CAD build for the part. Positions are in the model's coordinates, mm. A direction names the side the tool comes from. Coordinates: 2 decimals unless noted, no trailing zeros. Order: outer loops, then holes, each group sorted by start corner. A loop starts at its lowest first (then second) coordinate and runs counter-clockwise, first axis right, second up. Notation, with made-up numbers: M 0.25,-23 L 33.25,-23 A29 cw 33.25,4 Z; hole C 47,21.25 d3. An arc over 180 degrees is marked long. Write item = value, one per line.
from build123d import *

# Parameters (mm, degrees)
F0_W     = 28
F0_H     = 18
F0_W_2   = 21.8
F0_H_2   = 11.8
F1_DEPTH = 7
F2_W     = 35.8
F2_H     = 18
F2_W_2   = 21.8
F2_H_2   = 11.8
F3_DEPTH = 2
F4_W     = 7
F4_H     = 3
F5_DEPTH = 31.901
F6_SIZE  = 1.5


with BuildPart() as f1:
    # F0 (on Right) → F1 (new body)
    with BuildSketch(Plane.YZ):
        Rectangle(F0_W, F0_H)
        Rectangle(F0_W_2, F0_H_2, mode=Mode.SUBTRACT)
    extrude(amount=-F1_DEPTH)

    # F2 (on face) → F3 (join)
    with BuildSketch(Plane.YZ):
        Rectangle(F2_W, F2_H)
        Rectangle(F2_W_2, F2_H_2, mode=Mode.SUBTRACT)
    extrude(amount=F3_DEPTH)

    # F4 (on face) → F5 (cut, through all)
    with BuildSketch(Plane(origin=(0, 14, 0), x_dir=(-1, 0, 0), z_dir=(0, 1, 0))):
        with Locations((3.5, 0)):
            Rectangle(F4_W, F4_H)
    extrude(amount=-F5_DEPTH, mode=Mode.SUBTRACT)

    # F6
    f6_edges = [f1.edges().sort_by_distance(p)[0] for p in [
        (2, 17.9, 0),
        (2, 0, 9),
        (2, -17.9, 0),
        (2, 0, -9),
        (2, 0, 5.9),
        (2, 10.9, 0),
        (2, 0, -5.9),
        (2, -10.9, 0),
    ]]
    chamfer(f6_edges, length=F6_SIZE)


solid = f1.part
(1) Pull direction Y, two halves, no side cores. Call faces 6 (the face through (-3, -14, 5)), 7 (the face through (0, -16, 0)), 8 (the face through (-3, -10.9, 3)): +Y half, -Y half, draft (parallel to the pull), parting line (faces both ways), or undercut.
Evaluation:
face_6 = -Y half
face_7 = draft
face_8 = undercut
(2) Wall check: line 1 (Z direction, x = -5.25, y = -11); line 2 (Z direction, x = -2.5, y = -5); line 3 (Y direction, x = -1.5, z = -4.25). Give the ranges that are in metal, low to high. Write a range as from..to.
Evaluation:
line_1 = -9..-1.5, 1.5..9
line_2 = -9..-5.9, 5.9..9
line_3 = -14..-10.9, 10.9..14
(3) Slice it at D-D, the plane z = 0. Write the cut outline in (x, y).
Evaluation:
outline = M 0,-17.9 L 0.5,-17.9 L 2,-16.4 L 2,-12.4 L 0.5,-10.9 L 0,-10.9 Z; M 0,10.9 L 0.5,10.9 L 2,12.4 L 2,16.4 L 0.5,17.9 L 0,17.9 Z
(4) Slice it at C-C, the plane y = 6.5. Write the cut outline in (x, z), then the cut area to 3 significant figures.
Evaluation:
outline = M -7,-9 L 0.5,-9 L 2,-7.5 L 2,-7.4 L 0.5,-5.9 L -7,-5.9 Z; M -7,5.9 L 0.5,5.9 L 2,7.4 L 2,7.5 L 0.5,9 L -7,9 Z
area = 51.3 mm²
(5) Pin check, flat tips, straight feed: pin 1 Ø1.5 at (x, z) = (-5, -1) entering from -Y; pin 2 Ø2 at (x, z) = (-3, -4.5) entering from +Y. Stop position of each tip, or through.
Evaluation:
pin_1 = -14
pin_2 = 14
(6) Slice it at B-B, the plane x = -5.25. Write the cut outline in (y, z).
Evaluation:
outline = M -14,-9 L 14,-9 L 14,-1.5 L 10.9,-1.5 L 10.9,-5.9 L -10.9,-5.9 L -10.9,-1.5 L -14,-1.5 Z; M -14,1.5 L -10.9,1.5 L -10.9,5.9 L 10.9,5.9 L 10.9,1.5 L 14,1.5 L 14,9 L -14,9 Z
(7) Tool access for faces 1 (the face through (-3, 0, 5.9)), 2 (the face through (-7, 0, 7)), 3 (the face through (1.3, -0.2, 6.7)), 4 (the face through (-3, 14, -5)), 5 (the face through (-3, -12, -1.5)): list every direction of +Z, -Z, +X, -X, +Y, -Y with a clear straight run to the whole face (end or side of a thin tool).
Evaluation:
face_1 = +X, -X
face_2 = +Z, -Z, -X, +Y, -Y
face_3 = +X
face_4 = +Z, -Z, -X, +Y
face_5 = -X, +Y, -Y
(8) Slice it at A-A, the plane z = -3.5. Write the cut outline in (x, y).
Evaluation:
outline = M -7,-14 L 0,-14 L 0,-17.9 L 0.5,-17.9 L 2,-16.4 L 2,-12.4 L 0.5,-10.9 L -7,-10.9 Z; M -7,10.9 L 0.5,10.9 L 2,12.4 L 2,16.4 L 0.5,17.9 L 0,17.9 L 0,14 L -7,14 Z
